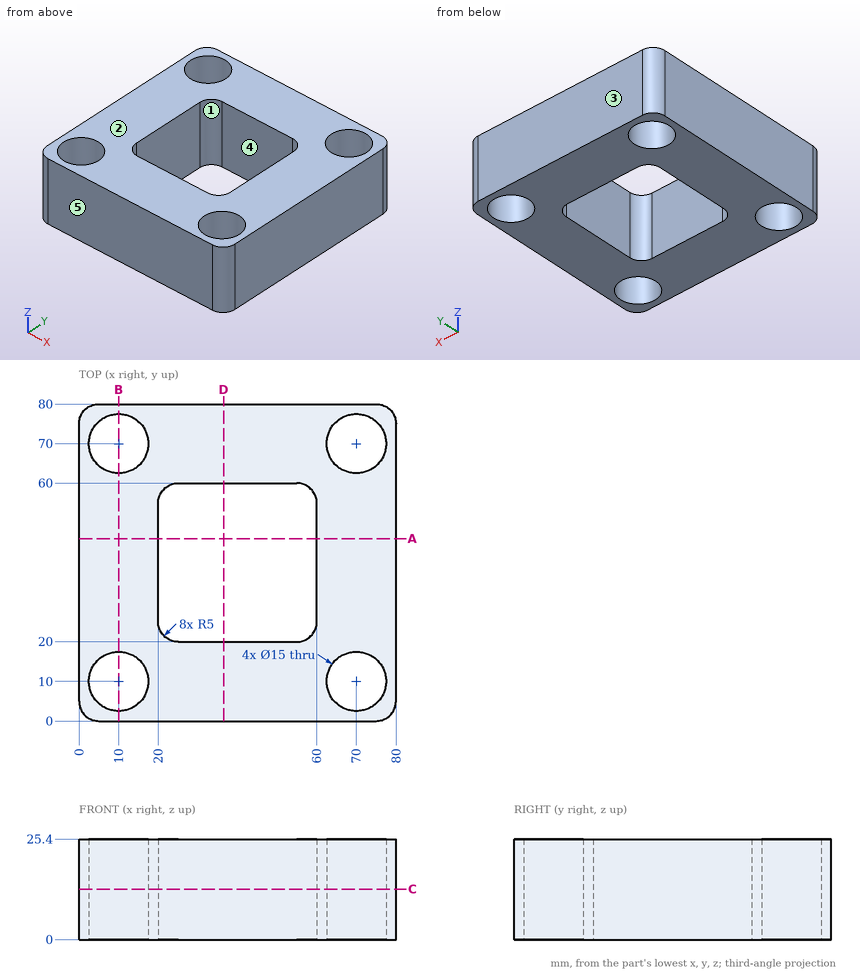
Source: three-view drawing plus pictorial views. Frame: mm from the lowest corner of the part. A direction names the side the tool comes from. Round coordinates to 2 decimals unless told otherwise and drop trailing zeros. Loops run counter-clockwise (first coordinate to the right, second up) from the corner with the lowest first, then second, coordinate; pieces in that order, holes last. Notation, with made-up numbers: M 40,9 L 87,9 A29 ccw 87,40 Z; hole C -4.5,48 d10. An arc over 180 degrees is marked long. Answer as CSV lines item,"result".
Q1. Cut plane C-C (z = 12.75). Return the cut outline in (x, y), plus the area to 3 significant figures.
Verdict:
outline,"M 0,5 A5 ccw 5,0 L 75,0 A5 ccw 80,5 L 80,75 A5 ccw 75,80 L 5,80 A5 ccw 0,75 Z; hole C 10,10 d15; hole C 10,70 d15; hole M 20,25 A5 ccw 25,20 L 55,20 A5 ccw 60,25 L 60,55 A5 ccw 55,60 L 25,60 A5 ccw 20,55 Z; hole C 70,10 d15; hole C 70,70 d15"
area,"4,090 mm^2"
Q2. Reachability of the marked faces 4 and 5 from +Z, -Z, +X, -X, +Y, -Y: full face, straight path, thin tool, end or side. Return the list, or none.
Verdict:
face 4,"+Z, -Z"
face 5,"+Z, -Z, +X, -X, -Y"
Q3. Line query: line 1 along Y through (x, z) = (70, 3.25); line 2 along X through (y, z) = (53, 6.25). Output: solid intervals per line, ascending.
Verdict:
line 1,"y = 0 to 2.5, 17.5 to 62.5, 77.5 to 80"
line 2,"x = 0 to 20, 60 to 80"
Q4. Pull-direction query (Y, two-part tool) for the marked faces 1, 2 and 3; classes: +Y half, -Y half, draft (parallel to the pull), parting line (faces both ways), or undercut.
Verdict:
face 1,"undercut"
face 2,"draft"
face 3,"+Y half"
Q5. Contact query for flat-ended pins moving along their axis: pin 1 (1 mm diameter, centred on x = 32.5, z = 6, fed in from -Y); pin 2 (9 mm diameter, centred on x = 70, y = 70, fed in from -Z). Output: stop coordinate, or through.
Verdict:
pin 1,"stops at y = 0"
pin 2,"passes through"
Q6. Cut plane B-B (x = 10). Return the cut outline in (y, z), plus the area to 3 significant figures.
Verdict:
outline,"M 0,0 L 2.5,0 L 2.5,25.4 L 0,25.4 Z; M 17.5,0 L 62.5,0 L 62.5,25.4 L 17.5,25.4 Z; M 77.5,0 L 80,0 L 80,25.4 L 77.5,25.4 Z"
area,"1,270 mm^2"
Q7. Cut plane A-A (y = 46). Return the cut outline in (x, z), plus the area to 3 significant figures.
Verdict:
outline,"M 0,0 L 20,0 L 20,25.4 L 0,25.4 Z; M 60,0 L 80,0 L 80,25.4 L 60,25.4 Z"
area,"1,020 mm^2"
